Read the model definition and answer for the solid it produces. Units are mm, in the model's axes. A direction names the side the tool comes from. Round coordinates to 2 decimals unless told otherwise and drop trailing zeros. Order: outer loops, then holes, each group sorted by start corner. A loop starts at its lowest first (then second) coordinate and runs counter-clockwise, first axis right, second up. Notation, with made-up numbers: (67, 16) - (126, 16) arc R17 ccw to (126, 45) - close; hole circle Ø2 at (63.25, 30). An arc over 180 degrees is marked (long way). Put each result on its own line as item: value. Start each with the question number.
Q1. Section D-D on x = 1.5 is taken. State how many separate pieces and enclosed holes the cut face has, then the cut area to 3 significant figures.
Q2. For a pull along X with two mould halves and no side action, classify faces 4 (the face through (1.5, 4.4, 3.5)), 5 (the face through (3.576, 0.864, 5.587)), 6 (the face through (3.74, 5.47, 9.53)) as pulls with the +X half, pulls with the -X half, needs draft (parallel to the pull), parting line crosses it, or undercut.
Q3. Section C-C on z = -1.75 is taken. Give the vertices of the cut face in (x, y) (3 decimals).
Q4. Section B-B on x = -1.5 is taken. Give the vertices of the cut face in (y, z) (3 decimals).
Q5. Find the intervals of material crossed by line 1 along Z through (x, y) = (-0.5, 7.75) (3 decimals); line 2 along X through (y, z) = (8, -2); line 3 along Z through (x, y) = (2, 1.5), in increasing order. Write a range as from..to.
Q6. Which of the six approach directions +Z, -Z, +X, -X, +Y, -Y give full straight-line access (tool end or side, diameter ignored) to faces 1 (the face through (0, 5, 10.795)), 2 (the face through (3.556, 7, 3)), 3 (the face through (3.57, 2.35, -6.73))?
Q7. Each of these flat-tipped pins is pushed along its axis until it touches: pin 1 Ø1 at (x, y) = (4, 1.5) entering from -Z; pin 2 Ø2 at (x, y) = (-3, 2.5) entering from +Z; pin 3 Ø1 at (y, z) = (2.24, -7.55) entering from +X. Where does it stop, or does it pass through?
Q8. Section A-A on y = 8 is taken. Give the vertices of the cut face in (x, z) (3 decimals), then the cut area to 3 significant figures.
Autodesk Inventor part; units mm, degrees
ref_plane "Work Plane1" through (0, 0, 0) normal (-1, 0, 0) x (0, 0, 1)
ref_plane "YZ Plane" through (0, 0, 0) normal (1, 0, 0) x (0, 1, 0)
ref_plane "XZ Plane" through (0, 0, 0) normal (0, 1, 0) x (-1, 0, 0)
sketch "Sketch1" plane through (0, 0, 0) normal (1, 0, 0) x (0, 1, 0)
  line L0 (0, 0) -> (0, 10.795)
  line L1 (0, 10.795) -> (10.795, 10.795)
  line L2 (10.795, 10.795) -> (10.795, 9.017)
  line L3 (10.795, 9.017) -> (5.8775, 9.017)
  line L4 (5.8775, 9.017) -> (3.81, 1.3008)
  line L5 (4.3488, 0.762) -> (10.795, 0.762)
  line L6 (10.795, 0.762) -> (10.795, 0)
  line L7 (0, 0) -> (10.795, 0) construction
  line L8 (3.81, 1.3008) -> (4.3488, 0.762)
  line L9 (0, 0) -> (0, -10.795)
  line L10 (0, -10.795) -> (10.795, -10.795)
  line L11 (10.795, -10.795) -> (10.795, -9.017)
  line L12 (10.795, -9.017) -> (5.8775, -9.017)
  line L13 (5.8775, -9.017) -> (3.81, -1.3008)
  line L14 (4.3488, -0.762) -> (10.795, -0.762)
  line L15 (10.795, -0.762) -> (10.795, 0)
  line L16 (3.81, -1.3008) -> (4.3488, -0.762)
  dimension "d0" = 10.795
  dimension "d1" = 105
  dimension "d8" = 0.762
  dimension "d33" = 3.81
  dimension "d34" = 10.795
  dimension "d35" = 0.762
  dimension "d36" = 1.778
extrude "Extrusion1" add sketch "Sketch1" along normal mid plane 7.112
sketch "Sketch2" plane through (3.556, 0, 0) normal (1, 0, 0) x (0, 0, -1)
  line L0 (-10.795, 10.795) -> (10.795, 10.795)
  line L1 (10.795, 10.795) -> (10.795, 0)
  line L2 (10.795, 0) -> (-10.795, 0)
  line L3 (-10.795, 0) -> (-10.795, 10.795)
  point P0 (0, 0)
extrude "Extrusion2" add sketch "Sketch2" along normal blind 1.524
ref_plane "Work Plane1" through (0, 0, 0) normal (-1, 0, 0) x (0, 0, 1)
mirror "Mirror1" about plane through (0, 0, 0) normal (-1, 0, 0) of "Extrusion2"
ref_plane "Work Plane2" through (3.556, 5.8775, 0) normal (0, 0, 1) x (1, 0, 0)
sketch "Sketch3" plane through (-3.556, 3.81, -1.3008) normal (0, 0.9659258, 0.258819) x (1, 0, 0)
  circle A0 centre (3.556, 4.4884) radius 2.286
  line L0 (3.556, -2.2426) -> (3.556, 4.4884) construction
  line L1 (7.112, 1.2874) -> (0, 1.2874) construction
  dimension "d14" = 4.572
  dimension "d15" = 6.731
extrude "Extrusion3" cut sketch "Sketch3" against normal blind 1.016
mirror "Mirror2" about plane through (3.556, 5.8775, 0) normal (0, 0, 1) of "Extrusion3"
fillet "Fillet4" radius 3.175 4 edges at (3.556, 8.3363, -9.017) (-3.556, 8.3363, -9.017) (3.556, 8.3363, 9.017) (-3.556, 8.3363, 9.017)
fillet "Fillet5" radius 4.445 4 edges at (5.08, 5.3975, 10.795) (5.08, 5.3975, -10.795) (-5.08, 5.3975, -10.795) (-5.08, 5.3975, 10.795)
sketch "Sketch4" plane through (0, 3.9903, 5.8992) normal (0, 0.9659258, -0.258819) x (1, 0, 0)
  line L0 (0, 0.0029) -> (0, -1.1401) construction
  line L1 (0, 0.0029) -> (0, 1.1459) construction
  line L2 (0, 0.0029) -> (0, -1.1079) construction
  circle A0 centre (0, 1.1459) radius 0.8255
  circle A1 centre (0, -1.1401) radius 0.8255
  line L3 (2.1143, 0.0029) -> (2.1143, 2.2658) construction
  point P0 (0, 6.731)
  dimension "d43" = 1.143
  dimension "d44" = 1.651
revolve "Revolution1" cut sketch "Sketch4" angle 90 about axis through (2.1143, 3.9896, 5.8964) along (0, 0.258819, 0.9659258)
mirror "Mirror3" about plane through (3.556, 5.8775, 0) normal (0, 0, 1) of "Revolution1"
sketch "Sketch6" plane through (2.1143, 4.7773, -7.6581) normal (-1, 0, 0) x (0, -1, 0)
  circle A0 centre (2.5341, 0.1105) radius 0.8255
  circle A1 centre (2.5341, 0.1105) radius 0.8255
  circle A2 centre (3.1258, 2.3186) radius 0.8255
  circle A3 centre (3.1258, 2.3186) radius 0.8255
  point P0 (4.7773, 7.6581)
extrude "Extrusion6" cut sketch "Sketch6" against normal up to next
mirror "Mirror10" about plane through (3.556, 5.8775, 0) normal (0, 0, 1) of "Extrusion6"
equation "\"d0\" = 0.5 * Base_Length"
equation "\"d1\" = Sensor_Angle"
equation "\"d33\" = Base_Thickness"
equation "\"d34\" = Mount_Height"
equation "\"d14\" = LED_Base"
equation "\"d15\" = Hole_to_Center"
equation "\"d18\" = Wire_Spacing"
equation "\"Wire_Spacing\" = 1.143"
equation "\"Wire_Diameter\" = 1.651"
equation "\"LED_Base\" = 4.572"
equation "\"Mount_Space\" = 16.51"
equation "\"Mount_Clearance\" = 3.175"
equation "\"Mount_Height\" = 10.795"
equation "\"Base_Length\" = 21.59"
equation "\"Base_Width\" = 10.16"
equation "\"Sensor_Angle\" = 105deg"
equation "\"Base_Thickness\" = 3.81"
equation "\"Hole_to_Center\" = 6.731"
equation "\"Tape_Width\" = 2.54"
properties part number "Line Tracker v3" material "PLA Plastic"
Findings:
1. separate pieces: 1
1. enclosed holes: 4
1. area: 118 mm2
2. face 4: undercut
2. face 5: needs draft
2. face 6: pulls with the +X half
3. outline: (-5.08, 0) - (5.08, 0) - (5.08, 10.795) - (3.556, 10.795) - (3.556, 3.93) - (-3.556, 3.93) - (-3.556, 10.795) - (-5.08, 10.795) - close
4. outline: (0, -10.71) - (10.795, -10.71) - (10.795, -8.813) - (5.823, -8.813) - (5.418, -7.303) - (4.435, -7.566) - (3.542, -4.233) - (4.525, -3.97) - (3.81, -1.301) - (4.349, -0.762) - (10.795, -0.762) - (10.795, 0.762) - (4.349, 0.762) - (3.81, 1.301) - (4.525, 3.97) - (3.542, 4.233) - (4.435, 7.566) - (5.418, 7.303) - (5.823, 8.813) - (10.795, 8.813) - (10.795, 10.71) - (0, 10.71) - close
5. line 1: -10.795..-9.015, -0.762..0.762, 9.015..10.795
5. line 2: -5.08..-3.56, 3.56..5.08
5. line 3: -10.58..-7.9, -7.19..-6.15, -4.53..4.53, 6.15..7.19, 7.9..10.58
6. face 1: +Z, +X, -X, +Y, -Y
6. face 2: +Y
6. face 3: +X
7. pin 1: z = -9.75
7. pin 2: z = 10.58
7. pin 3: x = 0.78
8. outline: (-5.08, -6.35) arc R4.445 ccw to (-0.635, -10.795) - (0.635, -10.795) arc R4.445 ccw to (5.08, -6.35) - (5.08, 6.35) arc R4.445 ccw to (0.635, 10.795) - (-0.635, 10.795) arc R4.445 ccw to (-5.08, 6.35) - close; hole (-3.556, -5.842) arc R3.175 ccw to (-0.381, -9.017) - (0.381, -9.017) arc R3.175 ccw to (3.556, -5.842) - (3.556, -0.762) - (-3.556, -0.762) - close; hole (-3.556, 0.762) - (3.556, 0.762) - (3.556, 5.842) arc R3.175 ccw to (0.381, 9.017) - (-0.381, 9.017) arc R3.175 ccw to (-3.556, 5.842) - close
8. area: 93.6 mm2
